Could you check a few things on this model? Use its own coordinates, in mm. Face numbers are marked on the shaded views. A direction names the side the tool comes from. Coordinates: 2 decimals unless noted, no trailing zeros. Loops run counter-clockwise (first coordinate to the right, second up) from the corner with the lowest first, then second, coordinate; pieces in that order, holes last.
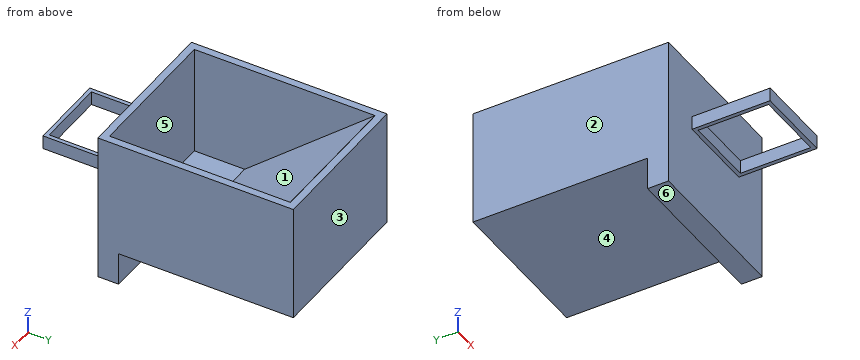
from build123d import *

# Parameters (mm, degrees)
F0_W      = 101.6
F0_H      = 76.2
F1_DEPTH  = 127
F2_T      = -4.7625
F4_DEPTH  = 101.6
F5_W      = 50.8
F5_H      = 8.89
F6_DEPTH  = 50.8
F7_W      = 45.72
F7_H      = 45.72
F8_DEPTH  = 25.4
F11_W     = 13.5890031233
F11_H     = 21.4630011469
F12_DEPTH = 101.6


# Not quite as in the source:
# - the program builds the solid bodies; features that only make, move or delete a surface that nothing else refers to are left out


with BuildPart() as f1:
    # F0 (on Front) → F1 (new body)
    with BuildSketch(Plane.XZ):
        with Locations((50.8, 38.1)):
            Rectangle(F0_W, F0_H)
    extrude(amount=-F1_DEPTH)

    # F2
    f2_openings = [f1.faces().sort_by_distance(p)[0] for p in [
        (50.8, 63.5, 76.2),
    ]]
    offset(amount=F2_T, openings=f2_openings)

    # F3 (on face) → F4 (join)
    with BuildSketch(Plane.YZ.offset(101.6)):
        Polygon((122.1133470535, 0), (122.1133470535, 76.2), (31.75, 0), align=None)
    extrude(amount=-F4_DEPTH)

    # F5 (on face) → F6 (join)
    with BuildSketch(Plane.XZ):
        with Locations((50.8, 36.195)):
            Rectangle(F5_W, F5_H)
    extrude(amount=F6_DEPTH)

    # F7 (on face) → F8 (cut)
    with BuildSketch(Plane.XY.offset(40.64)):
        with Locations((50.8, -25.4)):
            Rectangle(F7_W, F7_H)
    extrude(amount=-F8_DEPTH, mode=Mode.SUBTRACT)

    # F11 (on Right) → F12 (join)
    with BuildSketch(Plane.YZ):
        with Locations((6.7945015617, -10.7315005735)):
            Rectangle(F11_W, F11_H)
    extrude(amount=F12_DEPTH)


solid = f1.part
(1) For pin 1 (12 mm diameter, centred on x = 65.5, y = 63, fed in from -Z); pin 2 (10 mm diameter, centred on x = 48.5, y = 15, fed in from +Z); pin 3 (2.5 mm diameter, centred on y = -13, z = 36.5, fed in from +X), each with a flat end and sliding along its axis, tell me the tip position at first contact or that it passes through.
Answers:
pin 1: stops at z = 0
pin 2: stops at z = 4.76
pin 3: stops at x = 76.2
(2) We'd pull the mould along Y, two halves only. Please class the marked faces 1, 2 and 3: +Y half, -Y half, draft (parallel to the pull), parting line (faces both ways), or undercut.
Answers:
face 1: undercut
face 2: draft
face 3: +Y half
(3) Which directions (+Z, -Z, +X, -X, +Y, -Y) give clear straight access to the entire face, cutting with the end or side of a thin tool? Please do the marked faces 4, 5 and 6.
Answers:
face 4: -Z, +X, -X, +Y
face 5: +Z
face 6: -Z, +X, -X, +Y, -Y
(4) I need wall thicknesses on probe 1 along X at (y, z) = (41, 61.5); probe 2 along Z at (x, y) = (67, 14); probe 3 along Y at (x, z) = (70, -1). Which ranges of each line are inside material? Lowest first, please.
Answers:
probe 1: x = 0 to 4.76, 96.84 to 101.6
probe 2: z = 0 to 4.76
probe 3: y = 0 to 13.59
(5) Imagine slicing it at A-A, the plane x = 68.5. Write out the boundary of the cut face in (y, z), and give its area (3 significant figures).
Answers:
outline: (-50.8, 31.75) - (-48.26, 31.75) - (-48.26, 40.64) - (-50.8, 40.64) - close; (-2.54, 31.75) - (0, 31.75) - (0, -21.46) - (13.59, -21.46) - (13.59, 0) - (127, 0) - (127, 76.2) - (122.24, 76.2) - (122.24, 4.76) - (122.11, 4.76) - (122.11, 76.2) - (37.4, 4.76) - (4.76, 4.76) - (4.76, 76.2) - (0, 76.2) - (0, 40.64) - (-2.54, 40.64) - close
area: 4,650 mm2
(6) Imagine slicing it at C-C, the plane z = 23. Write out the boundary of the cut face in (x, y).
Answers:
outline: (0, 0) - (101.6, 0) - (101.6, 127) - (0, 127) - close; hole (4.76, 4.76) - (96.84, 4.76) - (96.84, 59.03) - (4.76, 59.03) - close; hole (4.76, 122.11) - (96.84, 122.11) - (96.84, 122.24) - (4.76, 122.24) - close
(7) Imagine slicing it at D-D, the plane y = 31. Write out the boundary of the cut face in (x, z), and give its area (3 significant figures).
Answers:
outline: (0, 0) - (101.6, 0) - (101.6, 76.2) - (96.84, 76.2) - (96.84, 4.76) - (4.76, 4.76) - (4.76, 76.2) - (0, 76.2) - close
area: 1,160 mm2
(8) Imagine slicing it at B-B, the plane y = -7. Write out the boundary of the cut face in (x, z).
Answers:
outline: (25.4, 31.75) - (27.94, 31.75) - (27.94, 40.64) - (25.4, 40.64) - close; (73.66, 31.75) - (76.2, 31.75) - (76.2, 40.64) - (73.66, 40.64) - close
